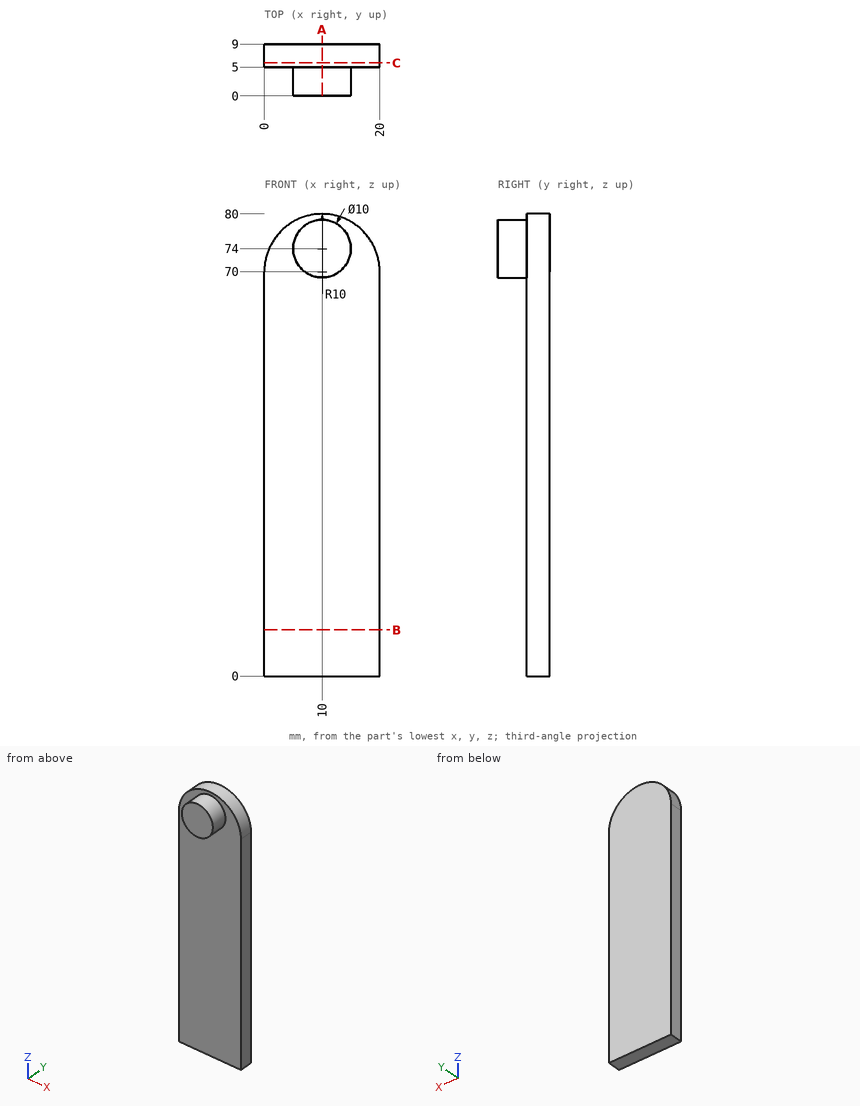
Answer from the drawing. Dimensions are ordinates in mm from the lowest x, y and z of the part. Round coordinates to 2 decimals unless told otherwise and drop trailing zeros. Order: outer loops, then holes, each group sorted by start corner. A loop starts at its lowest first (then second) coordinate and runs counter-clockwise, first axis right, second up.
1) The part is cut by section A-A on x = 10. Write down the section's boundary in (y, z).
2) Straight lines are drawn through the part: L1, parallel to Y at x = 18.5, z = 31; L2, parallel to Z at x = 9.75, y = 4.75; L3, parallel to Z at x = 4.75, y = 5.75. For each, find the intervals that lie inside material, in ascending order.
3) A flat-ended cylindrical pin translates along its axis: pin 1 (1 mm diameter, centred on x = 15, z = 71.5, fed in from -Y). Find the tip coordinate at first contact, or state that the pin passes through.
4) The part is cut by section B-B on z = 8. Write down the section's boundary in (x, y), plus the area to 3 significant figures.
5) The part is cut by section C-C on y = 5.75. Write down the section's boundary in (x, z).
Resolved:
1. outline: (0, 69) - (5, 69) - (5, 0) - (9, 0) - (9, 80) - (5, 80) - (5, 79) - (0, 79) - close
2. L1: y = 5 to 9
2. L2: z = 69.01 to 78.99
2. L3: z = 0 to 78.51
3. pin 1: stops at y = 5
4. outline: (0, 5) - (20, 5) - (20, 9) - (0, 9) - close
4. area: 80.0 mm2
5. outline: (0, 0) - (20, 0) - (20, 70) arc R10 ccw to (0, 70) - close
